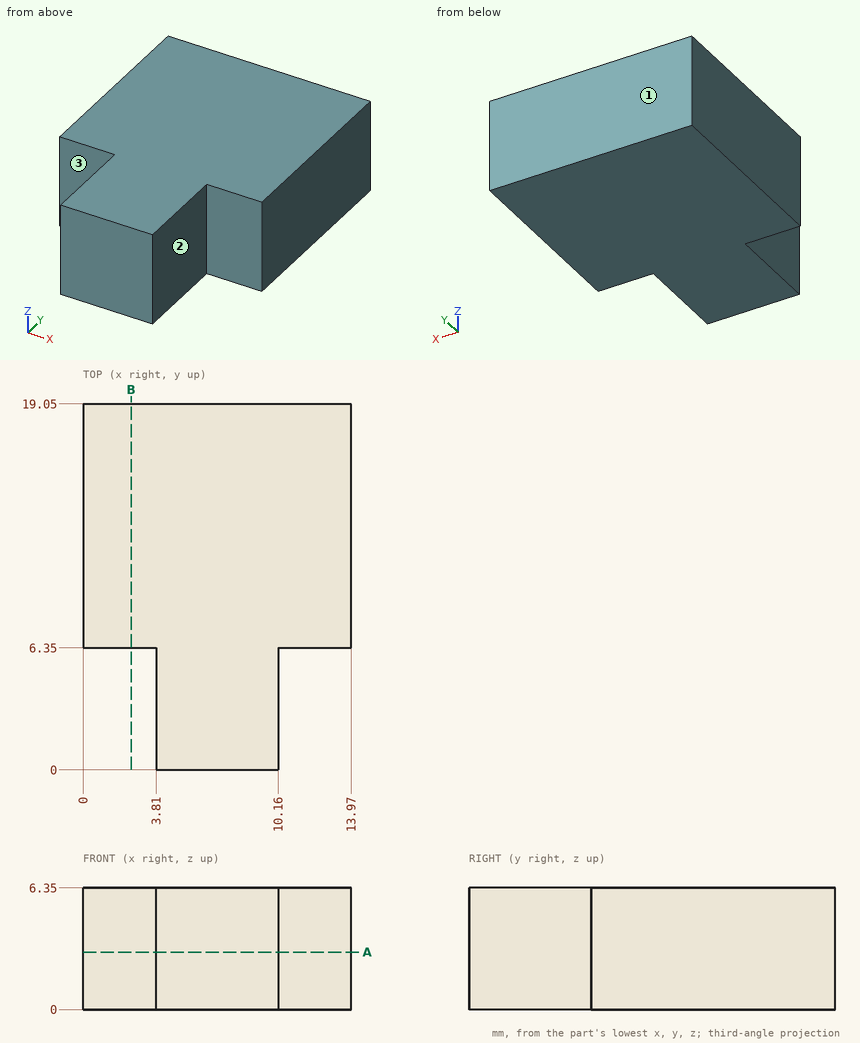
Geometry check sheet. Reference: drawing and pictorial views, mm from the part's lowest x, y, z. A direction names the side the tool comes from. Round coordinates to 2 decimals unless told otherwise and drop trailing zeros. Loops run counter-clockwise (first coordinate to the right, second up) from the corner with the lowest first, then second, coordinate; pieces in that order, holes last. Notation, with made-up numbers: (66, 20) - (106, 20) arc R19 cw to (106, 29) - close; hole circle Ø3 at (-35, 82.5). An arc over 180 degrees is marked (long way). Write item = value, one per line. Start each with the question number.
Q1. Depth check by flat-ended pin: P1, Ø3, axis at x = 13, z = 3, coming from the -Y side; P2, Ø1.9, axis at y = 4, z = 2, coming from the +X side; P3, Ø1.9, axis at y = 3, z = 3, coming from the -X side. Enter the tip coordinate at first touch or a pass-through.
Q2. Section check A-A (z = 3). Record the boundary of the cut face in (x, y), plus the area to 3 significant figures.
Q3. Section check B-B (x = 2.5). Record the boundary of the cut face in (y, z), plus the area to 3 significant figures.
Q4. Thickness scan on L1, parallel to Y at x = 3, z = 2.5; L2, parallel to X at y = 1.25, z = 1.75. Record the ranges inside material, lowest first.
Q5. Access from +Z, -Z, +X, -X, +Y, -Y to the whole of each face (thin tool, end or side, straight path). Record for the marked faces 1, 2 and 3.
Derived:
q1.P1 = 6.35
q1.P2 = 10.16
q1.P3 = 3.81
q2.outline = (0, 6.35) - (3.81, 6.35) - (3.81, 0) - (10.16, 0) - (10.16, 6.35) - (13.97, 6.35) - (13.97, 19.05) - (0, 19.05) - close
q2.area = 218 mm^2
q3.outline = (6.35, 0) - (19.05, 0) - (19.05, 6.35) - (6.35, 6.35) - close
q3.area = 80.6 mm^2
q4.L1 = 6.35 to 19.05
q4.L2 = 3.81 to 10.16
q5.face_1 = +Z, -Z, +X, -X, +Y
q5.face_2 = +Z, -Z, +X, -Y
q5.face_3 = +Z, -Z, -X, -Y
